Read the model definition and answer for the solid it produces. Units are mm, in the model's axes. A direction names the side the tool comes from. Coordinates: 2 decimals unless noted, no trailing zeros. Write each loop counter-clockwise with the first axis right and the second up, starting at its lowest first coordinate (ties: lowest second). Pieces come first, ordered by that corner, then holes. Notation, with made-up numbers: (70, 76) -> (115, 76) arc R23 cw to (115, 91) -> close; hole circle Ø4 at (4.5, 28). An arc over 180 degrees is marked (long way). Answer as a JSON object with one key per item and string values. Group by question number.
(1) Flat-ended cylindrical pins translate along their axes: P1, Ø5, axis at x = 9, y = 2.5, coming from the +Z side; P2, Ø2, axis at x = 1.5, y = 4, coming from the -Z side; P3, Ø1.9, axis at x = -4, z = -18.5, coming from the -Y side. Find the tip coordinate at first contact, or state that the pin passes through.
(2) Which of the six approach directions +Z, -Z, +X, -X, +Y, -Y give full straight-line access (tool end or side, diameter ignored) to faces 1 (the face through (0, 6.5, 19)), 2 (the face through (-1.7, 0, 15.3)), 3 (the face through (-19, 5, 0)), 4 (the face through (0, 3, -17.25)), 5 (the face through (21.25, 5, 0))?
(3) Find section B-B (y = 7). Give the vertices of the cut face in (x, z), then the cut area to 3 significant figures.
(4) Straight lines are drawn through the part: L1, parallel to X at y = 3.5, z = 13; L2, parallel to Z at x = 10.5, y = 4.5; L3, parallel to Z at x = 16, y = 7.5. For each, find the intervals that lie inside material, in ascending order.
(5) Find section C-C (z = -2.5). Give the vertices of the cut face in (x, y), then the cut area to 4 significant figures.
(6) For a pull along X with two mould halves and no side action, classify faces 6 (the face through (0, 8, -21)), 7 (the face through (0, 5, -15)), 8 (the face through (-21.25, 5, 0)), 9 (the face through (0, 5, 15)) as +X half, -X half, draft (parallel to the pull), parting line (faces both ways), or undercut.
(7) Find section D-D (y = 3). Give the vertices of the cut face in (x, z), then the cut area to 3 significant figures.
(8) Find section A-A (x = 16). Give the vertices of the cut face in (y, z), then the cut area to 4 significant figures.
from build123d import *

# Parameters (mm, degrees)
SKETCH_1_W      = 42.5
SKETCH_1_H      = 34.5
SKETCH_1_W_2    = 38
SKETCH_1_H_2    = 30
EXTRUDE_1_DEPTH = 6.5
SKETCH_2_W      = 42.5
SKETCH_2_H      = 42
SKETCH_2_W_2    = 38
SKETCH_2_H_2    = 30
EXTRUDE_2_DEPTH = 4


with BuildPart() as part:
    # Эскиз1 → Бобышка-Вытянуть1 (new body)
    with BuildSketch(Plane(origin=(0, 0, 0), x_dir=(1, 0, 0), z_dir=(0, 1, 0))):
        Rectangle(SKETCH_1_W, SKETCH_1_H)
        Rectangle(SKETCH_1_W_2, SKETCH_1_H_2, mode=Mode.SUBTRACT)
    extrude(amount=EXTRUDE_1_DEPTH)

    # Эскиз2 → Бобышка-Вытянуть2 (add)
    with BuildSketch(Plane(origin=(0, 6.5, 0), x_dir=(1, 0, 0), z_dir=(0, 1, 0))):
        Rectangle(SKETCH_2_W, SKETCH_2_H)
        Rectangle(SKETCH_2_W_2, SKETCH_2_H_2, mode=Mode.SUBTRACT)
    extrude(amount=EXTRUDE_2_DEPTH)


solid = part.part
Results below:
{
 "1": {"P1": "stops at z = 17.25", "P2": "stops at z = -17.25", "P3": "stops at y = 6.5"},
 "2": {"face 1": "+Z, +X, -X, -Y", "face 2": "+Z, -Z, +X, -X, -Y", "face 3": "+Y, -Y", "face 4": "-Z, +X, -X, -Y", "face 5": "+Z, -Z, +X, +Y, -Y"},
 "3": {"outline": "(-21.25, -21) -> (21.25, -21) -> (21.25, 21) -> (-21.25, 21) -> close; hole (-19, -15) -> (19, -15) -> (19, 15) -> (-19, 15) -> close", "area": "645 mm2"},
 "4": {"L1": "x = -21.25 to -19, 19 to 21.25", "L2": "z = -17.25 to -15, 15 to 17.25", "L3": "z = -21 to -15, 15 to 21"},
 "5": {"outline": "(-21.25, 0) -> (-19, 0) -> (-19, 10.5) -> (-21.25, 10.5) -> close; (19, 0) -> (21.25, 0) -> (21.25, 10.5) -> (19, 10.5) -> close", "area": "47.25 mm2"},
 "6": {"face 6": "draft", "face 7": "undercut", "face 8": "-X half", "face 9": "undercut"},
 "7": {"outline": "(-21.25, -17.25) -> (21.25, -17.25) -> (21.25, 17.25) -> (-21.25, 17.25) -> close; hole (-19, -15) -> (19, -15) -> (19, 15) -> (-19, 15) -> close", "area": "326 mm2"},
 "8": {"outline": "(0, -17.25) -> (6.5, -17.25) -> (6.5, -21) -> (10.5, -21) -> (10.5, -15) -> (0, -15) -> close; (0, 15) -> (10.5, 15) -> (10.5, 21) -> (6.5, 21) -> (6.5, 17.25) -> (0, 17.25) -> close", "area": "77.25 mm2"}
}
